Geometry: final body of the model. Coordinates: model frame, mm. A direction names the side the tool comes from. Coordinates: 2 decimals unless noted, no trailing zeros. Loops run counter-clockwise (first coordinate to the right, second up) from the corner with the lowest first, then second, coordinate; pieces in that order, holes last. Notation, with made-up numbers: (73, 15.5) - (96, 15.5) arc R18 cw to (96, 46.5) - close; hole circle Ø1 at (13, -16.75). An arc over 180 degrees is marked (long way). Put each result on its own line as item: value. Start each with the question number.
1) Section C-C on z = 22. Output: boundary loops of the cut face in (x, y), and give its area (3 significant figures).
2) Material intervals for line 1 along Z through (x, y) = (-4.45, 0); line 2 along X through (y, z) = (3, 17); line 3 along X through (y, z) = (-2.5, 18.5), sorted ascending. Write a range as from..to.
3) Contact query for flat-ended pins moving along their axis: pin 1 Ø2 at (x, z) = (-3.5, 13) entering from +Y; pin 2 Ø1 at (y, z) = (0.5, 8) entering from +X; pin 3 Ø5 at (y, z) = (2, 21.5) entering from -X. Output: stop coordinate, or through.
4) Section D-D on z = -46. Output: boundary loops of the cut face in (x, y), and give its area (3 significant figures).
5) Draft query along X for faces 1 (the flat face through (-2.476, 0, 21)), 2 (the flat face through (-4, 0, 29.312)), 3 (the cylindrical face through (-0.244, 5.545, -3.826)). Return one class per face: +X half, -X half, draft (parallel to the pull), parting line (faces both ways), or undercut.
6) Section A-A on y = 0. Output: boundary loops of the cut face in (x, z), and give its area (3 significant figures).
7) Section B-B on x = 0. Output: boundary loops of the cut face in (y, z), and give its area (3 significant figures).
8) Reachability of faces 4 (the cylindrical face through (3.99, 1.61, 25.56)), 5 (the cylindrical face through (-0.61, -1.95, -49.9)), 6 (the flat face through (2.476, 0, 21)) from +Z, -Z, +X, -X, +Y, -Y: full face, straight path, thin tool, end or side. Return the list, or none.
```python
from build123d import *

# Parameters (mm, degrees)
CUT_EXTRUDE4_DEPTH      = 5.5499
CUT_EXTRUDE4_DEPTH_BACK = 5.5499
SKETCH18_W              = 4.953
SKETCH18_H              = 17.526
CUT_EXTRUDE5_DEPTH      = 53.127561136
CUT_EXTRUDE5_DEPTH_BACK = 53.127561136
SKETCH19_R              = 1.6256


with BuildPart() as part:
    # Sketch17 → Revolve2 (revolve)
    with BuildSketch(Plane(origin=(0, 0, 0), x_dir=(0, 0, -1), z_dir=(1, 0, 0)), mode=Mode.PRIVATE) as revolve2_sk:
        Polygon((-29.3116, 0), (51.5112, 0), (51.5112, 2.0447), (48.3362, 2.0447), (48.3362, 5.6515), (37.6428, 5.6515), (37.6428, 5.5499), (-29.0576, 5.5499), (-29.3116, 5.2959), align=None)
    revolve(revolve2_sk.sketch.rotate(Axis((0, 0, 29.3116), (0, 0, -1)), 180), axis=Axis((0, 0, 29.3116), (0, 0, -1)))

    # Sketch18 → Cut-Extrude4 (cut, two sides: drawn at the far end of the back side and taken through both)
    with BuildSketch(Plane(origin=(0, 0, 0), x_dir=(1, 0, 0), z_dir=(0, 1, 0)).offset(-CUT_EXTRUDE4_DEPTH_BACK)):
        with Locations((0, -20.5486)):
            Rectangle(SKETCH18_W, SKETCH18_H)
    extrude(amount=CUT_EXTRUDE4_DEPTH + CUT_EXTRUDE4_DEPTH_BACK, mode=Mode.SUBTRACT)

    # Sketch19 → Cut-Extrude5 (cut, two sides: drawn at the far end of the back side and taken through both)
    with BuildSketch(Plane(origin=(0, 0, 0), x_dir=(0, 0, -1), z_dir=(1, 0, 0)).offset(-CUT_EXTRUDE5_DEPTH_BACK)):
        with Locations((-25.3492, 0)):
            Circle(SKETCH19_R)
    extrude(amount=CUT_EXTRUDE5_DEPTH + CUT_EXTRUDE5_DEPTH_BACK, mode=Mode.SUBTRACT)


solid = part.part
```
Answer block:
1. outline: (-2.48, -4.97) - (-2.48, 4.97) arc R5.55 ccw to start; (2.48, -4.97) arc R5.55 ccw to (2.48, 4.97) - close
1. area: 43.7 mm²
2. line 1: z = -48.34..23.72, 26.97..29.31
2. line 2: x = -4.67..-2.48, 2.48..4.67
2. line 3: x = -4.95..-2.48, 2.48..4.95
3. pin 1: stops at y = 4.95
3. pin 2: stops at x = 5.55
3. pin 3: stops at x = -5.55
4. outline: circle Ø11.3 at (0, 0)
4. area: 100 mm²
5. face 1: undercut
5. face 2: draft
5. face 3: parting line
6. outline: (-5.65, -48.34) - (-2.04, -48.34) - (-2.04, -51.51) - (2.04, -51.51) - (2.04, -48.34) - (5.65, -48.34) - (5.65, -37.64) - (5.55, -37.64) - (5.55, 23.72) - (2.48, 23.72) - (2.48, 11.79) - (-2.48, 11.79) - (-2.48, 23.72) - (-5.55, 23.72) - (-5.55, -37.64) - (-5.65, -37.64) - close; (-5.55, 26.97) - (-2.48, 26.97) - (-2.48, 29.31) - (-5.3, 29.31) - (-5.55, 29.06) - close; (2.48, 26.97) - (5.55, 26.97) - (5.55, 29.06) - (5.3, 29.31) - (2.48, 29.31) - close
6. area: 770 mm²
7. outline: (-5.65, -48.34) - (-2.04, -48.34) - (-2.04, -51.51) - (2.04, -51.51) - (2.04, -48.34) - (5.65, -48.34) - (5.65, -37.64) - (5.55, -37.64) - (5.55, 11.79) - (-5.55, 11.79) - (-5.55, -37.64) - (-5.65, -37.64) - close
7. area: 682 mm²
8. face 4: +X, -X
8. face 5: -Z
8. face 6: +Z, +Y, -Y
